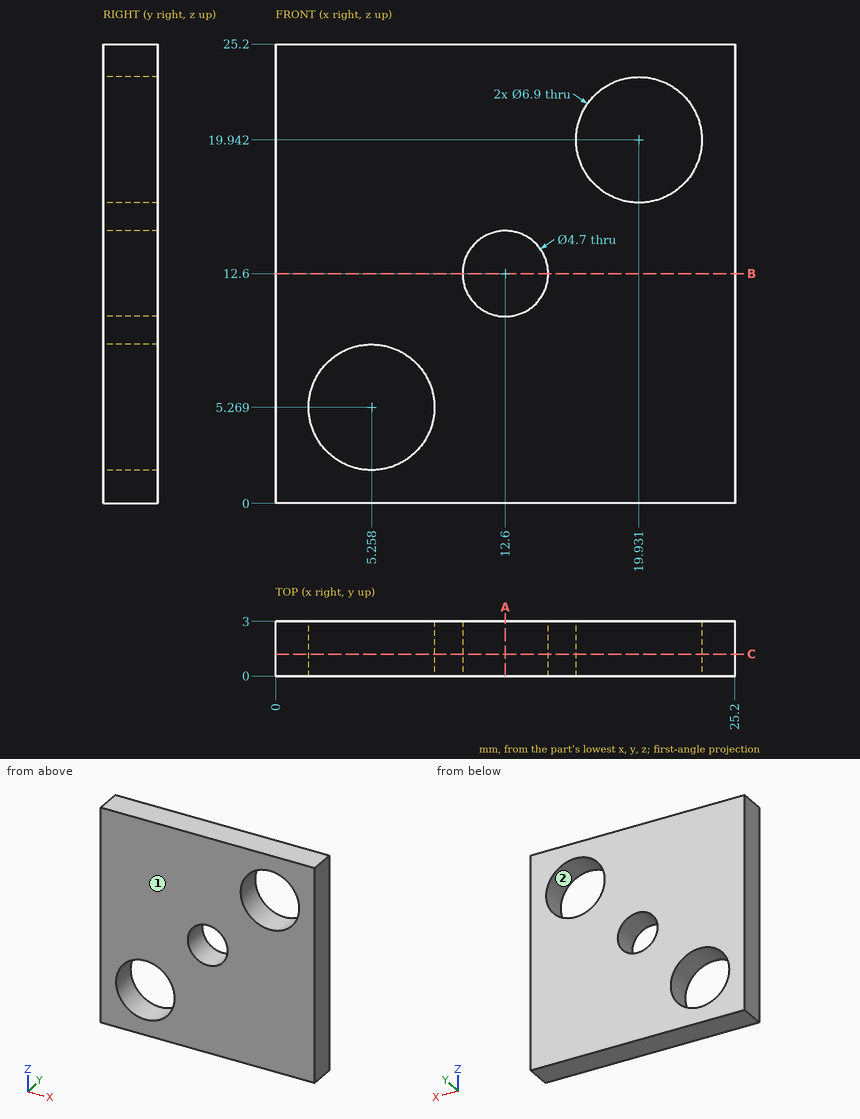
Can you work these out from the drawing? Everything is in mm from the part's minimum corner. Round coordinates to 2 decimals unless told otherwise and drop trailing zeros. Loops run counter-clockwise (first coordinate to the right, second up) from the corner with the lowest first, then second, coordinate; pieces in that order, holes last. Notation, with made-up numbers: (83.25, -30) -> (91.25, -30) arc R17 cw to (91.25, -9) -> close; hole circle Ø8 at (-16, 64). An arc over 180 degrees is marked (long way). Put each result on its own line as item: value.
Q1. I want a section at A-A on x = 12.6. Write out the boundary of the cut face in (y, z).
Checks:
outline: (0, 0) -> (3, 0) -> (3, 10.25) -> (0, 10.25) -> close; (0, 14.95) -> (3, 14.95) -> (3, 25.2) -> (0, 25.2) -> close
Q2. For pin 1 Ø4 at (x, z) = (5.26, 5.27) entering from +Y, with a flat end and sliding along its axis, tell me the tip position at first contact or that it passes through.
Checks:
pin 1: through
Q3. Please list where these lines run through material, in increasing order: line 1 (Z direction, x = 12.6, y = 1.95); line 2 (X direction, y = 2.8, z = 12.75) (1 decimal); line 3 (Z direction, x = 3.75, y = 2.15) (1 decimal). Write a range as from..to.
Checks:
line 1: 0..10.25, 14.95..25.2
line 2: 0..10.3, 14.9..25.2
line 3: 0..2.2, 8.4..25.2
Q4. I want a section at C-C on y = 1.2. Write out the boundary of the cut face in (x, z), and give its area (3 significant figures).
Checks:
outline: (0, 0) -> (25.2, 0) -> (25.2, 25.2) -> (0, 25.2) -> close; hole circle Ø6.9 at (5.26, 5.27); hole circle Ø4.7 at (12.6, 12.6); hole circle Ø6.9 at (19.93, 19.94)
area: 543 mm2
Q5. Thinking about a two-plate mould opening in X: for the marked faces 1 and 2, which applies, pulls with the +X half, pulls with the -X half, needs draft (parallel to the pull), parting line crosses it, or undercut?
Checks:
face 1: needs draft
face 2: undercut
Q6. I want a section at B-B on z = 12.6. Write out the boundary of the cut face in (x, y), and give its area (3 significant figures).
Checks:
outline: (0, 0) -> (10.25, 0) -> (10.25, 3) -> (0, 3) -> close; (14.95, 0) -> (25.2, 0) -> (25.2, 3) -> (14.95, 3) -> close
area: 61.5 mm2
